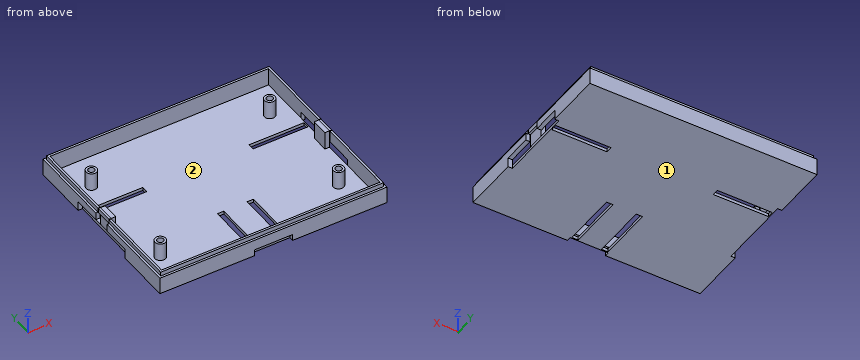
from build123d import *

# Parameters (mm, degrees)
SKETCH_W             = 107
SKETCH_H             = 87.7
SKETCH_R             = 1.5
SKETCH_W_2           = 3
SKETCH_H_2           = 26
SKETCH_W_3           = 26
SKETCH_H_3           = 3
PAD_DEPTH            = 10
SKETCH001_W          = 103
SKETCH001_H          = 83.7
SKETCH001_R          = 2.5
POCKET_DEPTH         = 8.5
SKETCH002_W          = 107
SKETCH002_H          = 87.7
SKETCH002_W_2        = 105
SKETCH002_H_2        = 85.7
POCKET001_DEPTH      = 2
SKETCH003_W          = 8.5
SKETCH003_H          = 8.5
POCKET002_DEPTH      = 53.501
POCKET002_DEPTH_BACK = 53.501
SKETCH004_W          = 18
SKETCH004_H          = 3
POCKET003_DEPTH      = 2
SKETCH005_W          = 35
SKETCH005_H          = 4.5
POCKET004_DEPTH      = 2
SKETCH006_W          = 35
SKETCH006_H          = 4.5
POCKET005_DEPTH      = 2
SKETCH007_W          = 2.120422
SKETCH007_H          = 8
PAD001_DEPTH         = 8.5
SKETCH008_W          = 7.99724
SKETCH008_H          = 2.093498
PAD002_DEPTH         = 1


with BuildPart() as part:
    # Sketch → Pad (new body)
    with BuildSketch(Plane.XY):
        Rectangle(SKETCH_W, SKETCH_H)
        with Locations((-42, -25.85)):
            Circle(SKETCH_R, mode=Mode.SUBTRACT)
        with Locations((42, 25.85)):
            Circle(SKETCH_R, mode=Mode.SUBTRACT)
        with Locations((-7, -28.35)):
            Rectangle(SKETCH_W_2, SKETCH_H_2, mode=Mode.SUBTRACT)
        with Locations((7, -28.35)):
            Rectangle(SKETCH_W_2, SKETCH_H_2, mode=Mode.SUBTRACT)
        with Locations((38, 12.85)):
            Rectangle(SKETCH_W_3, SKETCH_H_3, mode=Mode.SUBTRACT)
        with Locations((-38, 12.85)):
            Rectangle(SKETCH_W_3, SKETCH_H_3, mode=Mode.SUBTRACT)
    extrude(amount=PAD_DEPTH)

    # Sketch001 (on Face24 of Pad) → Pocket (cut)
    with BuildSketch(Plane.XY.offset(10)):
        Rectangle(SKETCH001_W, SKETCH001_H)
        with Locations((-42, -25.85)):
            Circle(SKETCH001_R, mode=Mode.SUBTRACT)
        with Locations((42, 25.85)):
            Circle(SKETCH001_R, mode=Mode.SUBTRACT)
    extrude(amount=-POCKET_DEPTH, mode=Mode.SUBTRACT)

    # Sketch002 (on Face5 of Pocket) → Pocket001 (cut)
    with BuildSketch(Plane.XY.offset(10)):
        Rectangle(SKETCH002_W, SKETCH002_H)
        Rectangle(SKETCH002_W_2, SKETCH002_H_2, mode=Mode.SUBTRACT)
    extrude(amount=-POCKET001_DEPTH, mode=Mode.SUBTRACT)

    # Sketch003 → Pocket002 (cut, two sides)
    with BuildSketch(Plane.YZ) as pocket002_sk:
        with Locations((0, 5.75)):
            Rectangle(SKETCH003_W, SKETCH003_H)
    extrude(amount=-POCKET002_DEPTH, mode=Mode.SUBTRACT)
    extrude(pocket002_sk.sketch, amount=POCKET002_DEPTH_BACK, mode=Mode.SUBTRACT)

    # Sketch004 (on Face1 of Pocket002) → Pocket003 (cut)
    with BuildSketch(Plane.XZ.offset(43.85)):
        with Locations((0, 1.5)):
            Rectangle(SKETCH004_W, SKETCH004_H)
    extrude(amount=-POCKET003_DEPTH, mode=Mode.SUBTRACT)

    # Sketch005 (on Face6 of Pocket003) → Pocket004 (cut)
    with BuildSketch(Plane.YZ.offset(53.5)):
        with Locations((0, 2.25)):
            Rectangle(SKETCH005_W, SKETCH005_H)
    extrude(amount=-POCKET004_DEPTH, mode=Mode.SUBTRACT)

    # Sketch006 (on Face8 of Pocket004) → Pocket005 (cut)
    with BuildSketch(Plane(origin=(-53.5, 0, 0), x_dir=(0, -1, 0), z_dir=(-1, 0, 0))):
        with Locations((0, 2.25)):
            Rectangle(SKETCH006_W, SKETCH006_H)
    extrude(amount=-POCKET005_DEPTH, mode=Mode.SUBTRACT)

    # Sketch007 (on Face49 of Pocket005) → Pad001 (join)
    with BuildSketch(Plane.XY.offset(1.5)):
        with Locations((-50.350937, 0.030608)):
            Rectangle(SKETCH007_W, SKETCH007_H)
    extrude(amount=PAD001_DEPTH)

    # Sketch008 (on Face64 of Pad001) → Pad002 (join)
    with BuildSketch(Plane(origin=(-51.411148, 0, 0), x_dir=(0, -1, 0), z_dir=(-1, 0, 0))):
        with Locations((-0.030066, 8.95208)):
            Rectangle(SKETCH008_W, SKETCH008_H)
    extrude(amount=PAD002_DEPTH)

    # Mirrored: part across YZ


with BuildPart() as part_1:
    add(part.part)
    add(part.part.mirror(Plane.YZ))


solid = part_1.part
The listing builds one solid part. Answer for the finished solid, in the listing's coordinates (mm). Face numbers are marked on the shaded views. Coordinates: 2 decimals unless noted, no trailing zeros. Loops run counter-clockwise (first coordinate to the right, second up) from the corner with the lowest first, then second, coordinate; pieces in that order, holes last. Notation, with made-up numbers: M 22,63 L 27,63 A23 cw 27,75 Z; hole C 16,35.25 d6. An arc over 180 degrees is marked long. Answer in a Markdown table with one row per item.
1) Given pin 1 (1 mm diameter, centred on x = 1, y = -26, fed in from +Z); pin 2 (1.6 mm diameter, centred on y = 19, z = 9, fed in from +X); pin 3 (2.5 mm diameter, centred on y = 0, z = 4.5, fed in from -X), each flat-ended and moving along its own axis, determine where each tip first touches the part or whether it passes through.
Answers below:
| item | result |
|---|---|
| pin 1 | z = 1.5 |
| pin 2 | x = 52.5 |
| pin 3 | x = -51.41 |
2) Find section A-A (y = 9.5). Determine the outline of the cut face in (x, z), then the cut area to 4 significant figures.
Answers below:
| item | result |
|---|---|
| outline | M -53.5,4.5 L -51.5,4.5 L -51.5,10 L -52.5,10 L -52.5,8 L -53.5,8 Z; M -51.5,0 L 51.5,0 L 51.5,1.5 L -51.5,1.5 Z; M 51.5,4.5 L 53.5,4.5 L 53.5,8 L 52.5,8 L 52.5,10 L 51.5,10 Z |
| area | 172.5 mm^2 |
3) Find section B-B (x = 2). Determine the outline of the cut face in (y, z), then the cut area to 3 significant figures.
Answers below:
| item | result |
|---|---|
| outline | M -43.85,3 L -41.85,3 L -41.85,10 L -42.85,10 L -42.85,8 L -43.85,8 Z; M -41.85,0 L 43.85,0 L 43.85,8 L 42.85,8 L 42.85,10 L 41.85,10 L 41.85,1.5 L -41.85,1.5 Z |
| area | 156 mm^2 |
4) Find section C-C (y = 29.5). Determine the outline of the cut face in (x, z).
Answers below:
| item | result |
|---|---|
| outline | M -53.5,0 L 53.5,0 L 53.5,8 L 52.5,8 L 52.5,10 L 51.5,10 L 51.5,1.5 L -51.5,1.5 L -51.5,10 L -52.5,10 L -52.5,8 L -53.5,8 Z |
5) Determine the mould class of the marked faces 1 and 2 for opening direction Y: released by +Y, released by -Y, zero draft, split by the parting line, or undercut.
Answers below:
| item | result |
|---|---|
| face 1 | zero draft |
| face 2 | undercut |
6) Find the intervals of material crossed by probe 1 along Y at (x, z) = (-42, 7.75); probe 2 along Y at (x, z) = (42, 8.25); probe 3 along X at (y, z) = (26, 4.25), in increasing order.
Answers below:
| item | result |
|---|---|
| probe 1 | -43.85 to -41.85, -28.35 to -27.35, -24.35 to -23.35, 23.35 to 24.35, 27.35 to 28.35, 41.85 to 43.85 |
| probe 2 | -42.85 to -41.85, -28.35 to -27.35, -24.35 to -23.35, 23.35 to 24.35, 27.35 to 28.35, 41.85 to 42.85 |
| probe 3 | -53.5 to -51.5, -44.5 to -43.49, -40.51 to -39.5, 39.5 to 40.51, 43.49 to 44.5, 51.5 to 53.5 |
